from build123d import *

# Parameters (mm, degrees)
EXTRUDE_1_DEPTH = 2


with BuildPart() as part:
    # 草图1 → 凸台-拉伸1 (new body)
    with BuildSketch(Plane(origin=(0, 0, 0), x_dir=(1, 0, 0), z_dir=(0, 1, 0))):
        with BuildLine():
            Line((31, 40.116685184), (-31, 40.116685184))
            ThreePointArc((-31, 40.116685184), (-34.535533906, 38.652219089), (-36, 35.116685184))
            Line((-36, 35.116685184), (-36, 5))
            ThreePointArc((-36, 5), (-34.535533906, 1.464466094), (-31, 0))
            Line((-31, 0), (31, 0))
            ThreePointArc((31, 0), (34.535533906, 1.464466094), (36, 5))
            Line((36, 5), (36, 35.116685184))
            ThreePointArc((36, 35.116685184), (34.535533906, 38.652219089), (31, 40.116685184))
        make_face()
        with BuildLine():
            Line((-31, 6.6), (0, 6.6))
            Line((0, 6.6), (31, 6.6))
            ThreePointArc((31, 6.6), (32.6, 5), (31, 3.4))
            Line((31, 3.4), (0, 3.4))
            Line((0, 3.4), (-31, 3.4))
            ThreePointArc((-31, 3.4), (-32.6, 5), (-31, 6.6))
        make_face(mode=Mode.SUBTRACT)
        with BuildLine():
            Line((-31, 16.6), (0, 16.6))
            Line((0, 16.6), (31, 16.6))
            ThreePointArc((31, 16.6), (32.6, 15), (31, 13.4))
            Line((31, 13.4), (0, 13.4))
            Line((0, 13.4), (-31, 13.4))
            ThreePointArc((-31, 13.4), (-32.6, 15), (-31, 16.6))
        make_face(mode=Mode.SUBTRACT)
        with BuildLine():
            Line((-31, 26.6), (0, 26.6))
            Line((0, 26.6), (31, 26.6))
            ThreePointArc((31, 26.6), (32.6, 25), (31, 23.4))
            Line((31, 23.4), (0, 23.4))
            Line((0, 23.4), (-31, 23.4))
            ThreePointArc((-31, 23.4), (-32.6, 25), (-31, 26.6))
        make_face(mode=Mode.SUBTRACT)
        with BuildLine():
            Line((-31, 36.6), (0, 36.6))
            Line((0, 36.6), (31, 36.6))
            ThreePointArc((31, 36.6), (32.6, 35), (31, 33.4))
            Line((31, 33.4), (0, 33.4))
            Line((0, 33.4), (-31, 33.4))
            ThreePointArc((-31, 33.4), (-32.6, 35), (-31, 36.6))
        make_face(mode=Mode.SUBTRACT)
    extrude(amount=EXTRUDE_1_DEPTH)


solid = part.part
Source: CAD feature listing. Evaluate the final solid. Frame: model axes, mm. A direction names the side the tool comes from. Round coordinates to 2 decimals unless told otherwise and drop trailing zeros. Loops run counter-clockwise (first coordinate to the right, second up) from the corner with the lowest first, then second, coordinate; pieces in that order, holes last. Notation, with made-up numbers: M 8,51.5 L 26,51.5 A19 cw 26,72.5 Z; hole C -29,-37 d6. An arc over 180 degrees is marked long. Return JSON: item names as keys, results as strings. Group by question number.
1. Reachability of faces 1 (the face through (0, 1, -16.6)), 2 (the face through (34, 1, -1)) from +Z, -Z, +X, -X, +Y, -Y: full face, straight path, thin tool, end or side. Return the list, or none.
2. Pin query (flat end, axial travel): pin 1 (2 mm diameter, centred on x = -11, z = -9, fed in from -Y). Return the tip coordinate at first contact, or that it passes through.
3. Mould query, pull axis Z, two halves, no side actions, for faces 3 (the face through (34.574, 0.986, -38.613)), 4 (the face through (32.6, 1, -5)), 5 (the face through (-1, 2, -20)). Classes: released by +Z, released by -Z, zero draft, split by the parting line, or undercut.
4. Section query B-B on x = 7. Output: boundary loops of the cut face in (y, z), and give its area (3 significant figures).
5. Section query C-C on y = 1.05. Output: boundary loops of the cut face in (x, z), and give its area (3 significant figures).
6. Section query A-A on z = -25. Output: boundary loops of the cut face in (x, y), and give its area (3 significant figures).
7. Material intervals for line 1 along Z through (x, y) = (24, 1.7); line 2 along X through (y, z) = (1.35, -24); line 3 along X through (y, z) = (1.8, -4), sorted ascending. Write a range as from..to.
Checks:
{
 "1": {"face 1": "+Y, -Y", "face 2": "+Z, +X, +Y, -Y"},
 "2": {"pin 1": "stops at y = 0"},
 "3": {"face 3": "released by -Z", "face 4": "undercut", "face 5": "zero draft"},
 "4": {"outline": "M 0,-40.12 L 2,-40.12 L 2,-36.6 L 0,-36.6 Z; M 0,-33.4 L 2,-33.4 L 2,-26.6 L 0,-26.6 Z; M 0,-23.4 L 2,-23.4 L 2,-16.6 L 0,-16.6 Z; M 0,-13.4 L 2,-13.4 L 2,-6.6 L 0,-6.6 Z; M 0,-3.4 L 2,-3.4 L 2,0 L 0,0 Z", "area": "54.6 mm²"},
 "5": {"outline": "M -36,-35.12 A5 ccw -31,-40.12 L 31,-40.12 A5 ccw 36,-35.12 L 36,-5 A5 ccw 31,0 L -31,0 A5 ccw -36,-5 Z; hole M -31,-36.6 L 31,-36.6 A1.6 ccw 31,-33.4 L -31,-33.4 A1.6 ccw Z; hole M -31,-26.6 L 31,-26.6 A1.6 ccw 31,-23.4 L -31,-23.4 A1.6 ccw Z; hole M -31,-16.6 L 31,-16.6 A1.6 ccw 31,-13.4 L -31,-13.4 A1.6 ccw Z; hole M -31,-6.6 L 31,-6.6 A1.6 ccw 31,-3.4 L -31,-3.4 A1.6 ccw Z", "area": "2,040 mm²"},
 "6": {"outline": "M -36,0 L -32.6,0 L -32.6,2 L -36,2 Z; M 32.6,0 L 36,0 L 36,2 L 32.6,2 Z", "area": "13.6 mm²"},
 "7": {"line 1": "z = -40.12..-36.6, -33.4..-26.6, -23.4..-16.6, -13.4..-6.6, -3.4..0", "line 2": "x = -36..-32.25, 32.25..36", "line 3": "x = -35.9..-32.25, 32.25..35.9"}
}
